Part print with two shaded views. Sizes in mm from the minimum x, y, z corner. A direction names the side the tool comes from. Give positions to 0.01 mm unless a question says otherwise; leave off trailing zeros. Write each loop counter-clockwise with the first axis right and the second up, starting at its lowest first coordinate (ties: lowest second). Pieces come first, ordered by that corner, then holes. Notation, with made-up numbers: M 45,-13.5 L 103,-13.5 A23 ccw 103,-5.5 Z; hole C -27.5,-29 d9. An arc over 180 degrees is marked long. Return JSON: item names as keys, results as strings. Group by question number.
Q1. Band-saw the part on D-D, the plane y = 199. Give the cut face in (x, z).
Q2. Band-saw the part on A-A, the plane z = 121. Give the cut face in (x, y).
Q3. Tool access for the marked faces 1, 2 and 3: list every direction of +Z, -Z, +X, -X, +Y, -Y with a clear straight run to the whole face (end or side of a thin tool).
Q4. Band-saw the part on C-C, the plane y = 234.5. Give the cut face in (x, z).
Q5. Pull direction Y, two halves, no side cores. Call the marked faces 4, 5, 6 and 7: +Y half, -Y half, draft (parallel to the pull), parting line (faces both ways), or undercut.
Q6. Band-saw the part on B-B, the plane x = 13.5. Give the cut face in (y, z), then the cut area to 3 significant figures.
Q7. Flat gauge pins, fed straight in: pin 1 Ø6 at (x, z) = (12, 131) entering from -Y; pin 2 Ø6 at (x, z) = (15, 127.5) entering from +Y; pin 3 Ø10 at (x, y) = (11, 36.5) entering from +Z; pin 4 Ø1.5 at (y, z) = (33.5, 71) entering from -X. Where does each tip first touch, or does it go through?
Q8. Wall check: probe 1 along Y at (x, z) = (5, 121); probe 2 along Z at (x, y) = (4.25, 16.5); probe 3 along Z at (x, y) = (8, 165). Give the ranges that are in metal, low to high.
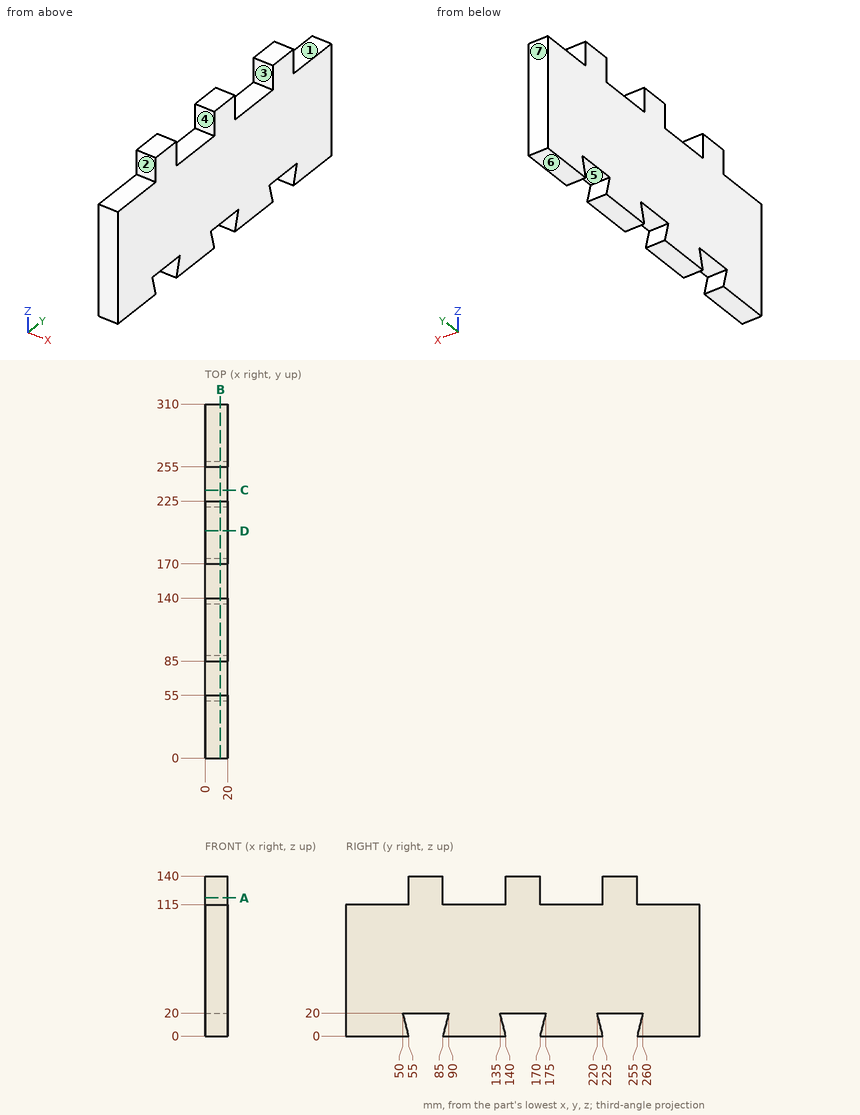
From the geometry:
{
 "1": {"outline": "M 0,0 L 20,0 L 20,115 L 0,115 Z"},
 "2": {"outline": "M 0,55 L 20,55 L 20,85 L 0,85 Z; M 0,140 L 20,140 L 20,170 L 0,170 Z; M 0,225 L 20,225 L 20,255 L 0,255 Z"},
 "3": {"face 1": "+Z, +X, -X, +Y", "face 2": "+Z, +X, -X, -Y", "face 3": "+Z, +X, -X"},
 "4": {"outline": "M 0,20 L 20,20 L 20,140 L 0,140 Z"},
 "5": {"face 4": "undercut", "face 5": "undercut", "face 6": "draft", "face 7": "+Y half"},
 "6": {"outline": "M 0,0 L 55,0 L 50,20 L 90,20 L 85,0 L 140,0 L 135,20 L 175,20 L 170,0 L 225,0 L 220,20 L 260,20 L 255,0 L 310,0 L 310,115 L 255,115 L 255,140 L 225,140 L 225,115 L 170,115 L 170,140 L 140,140 L 140,115 L 85,115 L 85,140 L 55,140 L 55,115 L 0,115 Z", "area": "35,800 mm^2"},
 "7": {"pin 1": "stops at y = 55", "pin 2": "stops at y = 255", "pin 3": "stops at z = 115", "pin 4": "stops at x = 0"},
 "8": {"probe 1": "y = 55 to 85, 140 to 170, 225 to 255", "probe 2": "z = 0 to 115", "probe 3": "z = 20 to 140"}
}
